Geometry: final body of the model. Coordinates: model frame, mm. A direction names the side the tool comes from. Round coordinates to 2 decimals unless told otherwise and drop trailing zeros. Loops run counter-clockwise (first coordinate to the right, second up) from the corner with the lowest first, then second, coordinate; pieces in that order, holes last. Notation, with made-up numbers: M -3.5,48.5 L 34.5,48.5 A6 cw 34.5,54.5 Z; hole C 57.5,88.25 d11. An arc over 180 degrees is marked long. Answer as a JSON object with one key per item and string values.
from build123d import *

# Parameters (mm, degrees)
SKETCH1_W                = 84.3
SKETCH1_H                = 85.09
BOSS_EXTRUDE1_DEPTH      = 1.6
SKETCH2_W                = 67.5
SKETCH2_H                = 51.5
BOSS_EXTRUDE2_DEPTH      = 3.1
CUT_EXTRUDE1_DEPTH       = 120.818229414
BOSS_EXTRUDE3_DEPTH      = 8
BOSS_EXTRUDE3_DEPTH_BACK = 10.4
SKETCH4_W                = 23.36
SKETCH4_H                = 5
SKETCH4_W_2              = 36.06


with BuildPart() as part:
    # Sketch1 → Boss-Extrude1 (new body)
    with BuildSketch(Plane.XY):
        with Locations((42.15, -42.545)):
            Rectangle(SKETCH1_W, SKETCH1_H)
    extrude(amount=BOSS_EXTRUDE1_DEPTH)

    # Sketch2 → Boss-Extrude2 (add)
    with BuildSketch(Plane.XY.offset(1.6)):
        with Locations((41.55, -39.05)):
            Rectangle(SKETCH2_W, SKETCH2_H)
    extrude(amount=BOSS_EXTRUDE2_DEPTH)

    # Sketch3 → Cut-Extrude1 (cut, through all)
    with BuildSketch(Plane.XY.offset(1.6)):
        Polygon((84.3, 0), (58.4, 0), (58.4, -5.8), (74.7, -5.8), (74.7, -10.89), (84.3, -10.89), align=None)
    extrude(amount=-CUT_EXTRUDE1_DEPTH, mode=Mode.SUBTRACT)

    # Sketch4 → Boss-Extrude3 (add, two sides: drawn at the far end of the back side and taken through both)
    with BuildSketch(Plane.XY.offset(1.6).offset(-BOSS_EXTRUDE3_DEPTH_BACK)):
        with Locations((28.98, -76.49)):
            Rectangle(SKETCH4_W, SKETCH4_H)
        with Locations((61.57, -76.49)):
            Rectangle(SKETCH4_W_2, SKETCH4_H)
        with Locations((34.13, -5.8)):
            Rectangle(SKETCH4_W_2, SKETCH4_H)
    extrude(amount=BOSS_EXTRUDE3_DEPTH + BOSS_EXTRUDE3_DEPTH_BACK)


solid = part.part
1) Ray query, line 1 (Y direction, x = 60.5, z = 3); line 2 (X direction, y = -76, z = -3.75); line 3 (Y direction, x = 23, z = -5.5). Return the intervals inside material, ascending.
Results:
{"line 1": "-78.99 to -73.99, -64.8 to -13.3", "line 2": "17.3 to 40.66, 43.54 to 79.6", "line 3": "-78.99 to -73.99, -8.3 to -3.3"}
2) Pin query (flat end, axial travel): P1, Ø1.5, axis at x = 75, y = -59, coming from the +Z side; P2, Ø8, axis at x = 22.5, z = -1.5, coming from the +Y side; P3, Ø2.5, axis at x = 29, z = -3.5, coming from the +Y side; P4, Ø2.5, axis at y = -6, z = 7.5, coming from the +X side. Return the tip coordinate at first contact, or that it passes through.
Results:
{"P1": "z = 4.7", "P2": "y = 0", "P3": "y = -3.3", "P4": "x = 52.16"}
3) Section query B-B (x = 35). Return the cut outline in (y, z), and give its area (3 significant figures).
Results:
{"outline": "M -85.09,0 L -78.99,0 L -78.99,-8.8 L -73.99,-8.8 L -73.99,0 L -8.3,0 L -8.3,-8.8 L -3.3,-8.8 L -3.3,0 L 0,0 L 0,1.6 L -3.3,1.6 L -3.3,9.6 L -8.3,9.6 L -8.3,1.6 L -13.3,1.6 L -13.3,4.7 L -64.8,4.7 L -64.8,1.6 L -73.99,1.6 L -73.99,9.6 L -78.99,9.6 L -78.99,1.6 L -85.09,1.6 Z", "area": "464 mm2"}
4) Section query C-C (y = -60). Return the cut outline in (x, z).
Results:
{"outline": "M 0,0 L 84.3,0 L 84.3,1.6 L 75.3,1.6 L 75.3,4.7 L 7.8,4.7 L 7.8,1.6 L 0,1.6 Z"}
5) Pull-direction query (X, two-part tool) for faces 5 (the flat face through (41, -64.8, 3)), 6 (the flat face through (43.54, -77, 6)), 7 (the flat face through (79.6, -77, -4)), 8 (the flat face through (43.54, -77, -4)); classes: +X half, -X half, draft (parallel to the pull), parting line (faces both ways), or undercut.
Results:
{"face 5": "draft", "face 6": "undercut", "face 7": "+X half", "face 8": "undercut"}
6) Reachability of faces 1 (the flat face through (34, -3.3, 6)), 2 (the flat face through (61, -78.99, 6)), 3 (the flat face through (40.66, -77, 6)), 4 (the flat face through (34, -8.3, -4)) from +Z, -Z, +X, -X, +Y, -Y: full face, straight path, thin tool, end or side. Return the list, or none.
Results:
{"face 1": "+Z, +X, -X, +Y", "face 2": "+Z, +X, -X, -Y", "face 3": "+Z, -Y", "face 4": "-Z, +X, -X"}
7) Section query A-A (z = -3.75). Return the cut outline in (x, y), and give its area (3 significant figures).
Results:
{"outline": "M 16.1,-8.3 L 52.16,-8.3 L 52.16,-3.3 L 16.1,-3.3 Z; M 17.3,-78.99 L 40.66,-78.99 L 40.66,-73.99 L 17.3,-73.99 Z; M 43.54,-78.99 L 79.6,-78.99 L 79.6,-73.99 L 43.54,-73.99 Z", "area": "477 mm2"}
8) Section query D-D (x = 76.5). Return the cut outline in (y, z), and give its area (3 significant figures).
Results:
{"outline": "M -85.09,0 L -78.99,0 L -78.99,-8.8 L -73.99,-8.8 L -73.99,0 L -10.89,0 L -10.89,1.6 L -73.99,1.6 L -73.99,9.6 L -78.99,9.6 L -78.99,1.6 L -85.09,1.6 Z", "area": "203 mm2"}
